Drawing for the job (mm, zero at the part's lowest x, y, z). A direction names the side the tool comes from. Give positions to 0.01 mm unless a question says otherwise; leave off trailing zeros. Order: outer loops, then holes, each group sorted by start corner. A loop starts at its lowest first (then second) coordinate and runs counter-clockwise, first axis right, second up. Notation, with made-up numbers: (11, 32.5) - (40, 32.5) arc R18 ccw to (40, 48.5) - close; hole circle Ø7 at (57.25, -20). An arc over 180 degrees is marked (long way). One line per item, written item: value.
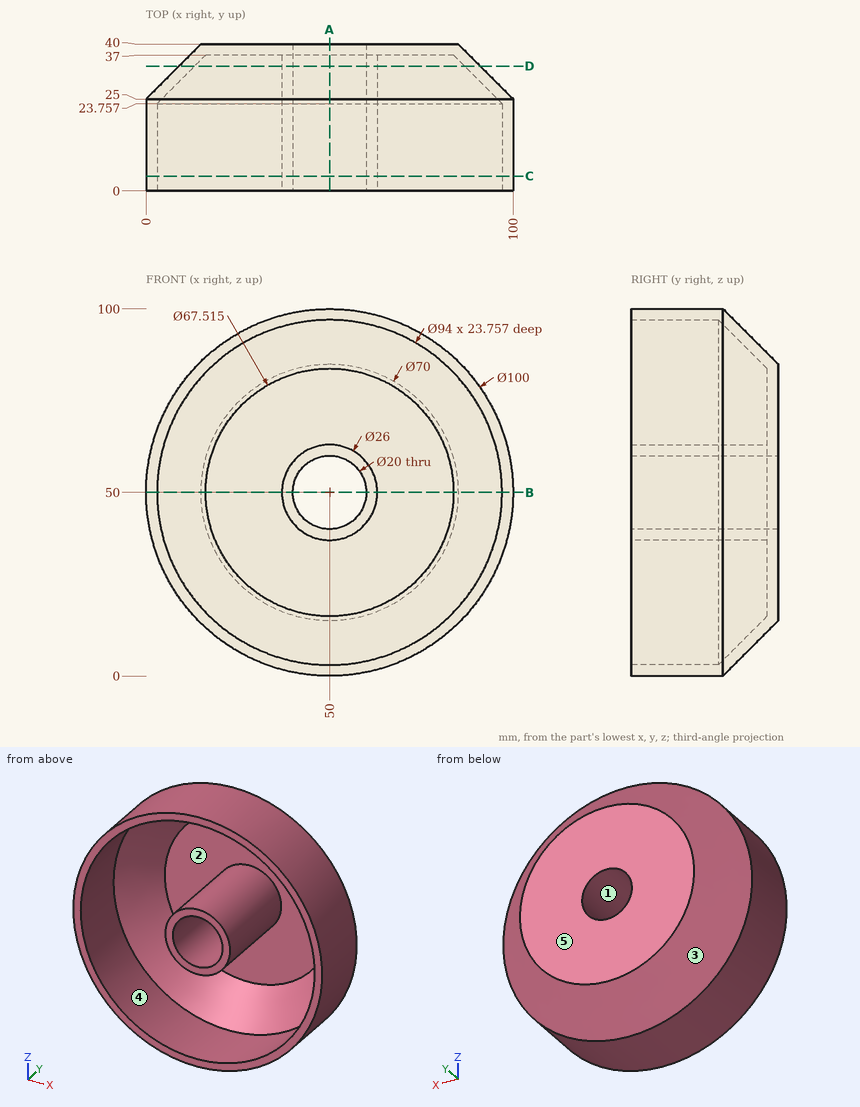
(1) Drill centre lines: line 1 (X direction, y = 21, z = 50); line 2 (Z direction, x = 58, y = 36.5) (1 decimal); line 3 (Z direction, x = 38, y = 22) (1 decimal). Where is each one in solid material? Low to high.
Completed:
line 1: 0 to 3, 37 to 40, 60 to 63, 97 to 100
line 2: 12.3 to 16.7, 39.8 to 44, 56 to 60.2, 83.3 to 87.7
line 3: 1.5 to 4.6, 45 to 55, 95.4 to 98.5
(2) Pin check, flat tips, straight feed: P1, Ø8, axis at x = 38, y = 20, coming from the +Z side; P2, Ø3, axis at x = 13, y = 15, coming from the +Z side; P3, Ø2, axis at x = 20.5, y = 25, coming from the +Z side; P4, Ø20.5, axis at x = 39, z = 33.5, coming from the -Y side. Stop position of each tip, or through.
Completed:
P1: z = 99.36
P2: z = 85.21
P3: z = 91.08
P4: y = 0
(3) 3-axis set-ups, long thin cutter, end or side, ignore diameter. For the marked faces 1 and 2: which of +Z, -Z, +X, -X, +Y, -Y reach the whole face in a straight line?
Completed:
face 1: +Y, -Y
face 2: -Y
(4) Pull direction Z, two halves, no side cores. Call the marked faces 3, 4 and 5: +Z half, -Z half, draft (parallel to the pull), parting line (faces both ways), or undercut.
Completed:
face 3: parting line
face 4: undercut
face 5: draft
(5) Slice it at B-B, the plane z = 50. Give the cut face in (x, y).
Completed:
outline: (0, 0) - (3, 0) - (3, 23.76) - (16.24, 37) - (37, 37) - (37, 0) - (40, 0) - (40, 40) - (15, 40) - (0, 25) - close; (60, 0) - (63, 0) - (63, 37) - (83.76, 37) - (97, 23.76) - (97, 0) - (100, 0) - (100, 25) - (85, 40) - (60, 40) - close
(6) Slice it at C-C, the plane y = 4. Give the cut face in (x, z), and give its area (3 significant figures).
Completed:
outline: circle Ø100 at (50, 50); circle Ø26 at (50, 50); hole circle Ø94 at (50, 50); hole circle Ø20 at (50, 50)
area: 1,130 mm²
(7) Slice it at A-A, the plane x = 50. Give the cut face in (y, z).
Completed:
outline: (0, 0) - (25, 0) - (40, 15) - (40, 40) - (0, 40) - (0, 37) - (37, 37) - (37, 16.24) - (23.76, 3) - (0, 3) - close; (0, 60) - (40, 60) - (40, 85) - (25, 100) - (0, 100) - (0, 97) - (23.76, 97) - (37, 83.76) - (37, 63) - (0, 63) - close
(8) Slice it at D-D, the plane y = 34. Give the cut face in (x, z) (1 decimal).
Completed:
outline: circle Ø82 at (50, 50); circle Ø26 at (50, 50); hole circle Ø73.5 at (50, 50); hole circle Ø20 at (50, 50)
